Print and shaded views of the part. All mm, measured from the part's lowest x, y and z. Give positions to 0.01 mm unless a question says otherwise; leave off trailing zeros. Order: outer loops, then holes, each group sorted by start corner. A loop starts at its lowest first (then second) coordinate and runs counter-clockwise, first axis right, second up. Notation, with made-up numbers: (15, 78) -> (36, 78) arc R34 ccw to (36, 113) -> close; hole circle Ø11 at (-29, 36). An arc over 180 degrees is marked (long way). One line per question, with ' | ' between items. Start each with the question number.
(1) Cut at B-B (y = 1.35). Give the cut face in (x, z), then the cut area to 3 significant figures.
(2) Cut at A-A (x = 103.5). Give the cut face in (y, z), then the cut area to 4 significant figures.
(3) Cut at C-C (z = 39.5). Give the cut face in (x, y), then the cut area to 4 significant figures.
(4) Pin check, flat tips, straight feed: pin 1 Ø1.1 at (y, z) = (1.5, 19.5) entering from +X; pin 2 Ø0.5 at (x, y) = (96.5, 1.5) entering from -Z; pin 3 Ø0.5 at (y, z) = (1.5, 40.5) entering from -X. Stop position of each tip, or through.
(5) Drill centre lines: L1, parallel to Z at x = 112, y = 1.2; L2, parallel to X at y = 1.55, z = 23.5; L3, parallel to X at y = 0.8, z = 2. Where is each one in solid material? Low to high. Write a range as from..to.
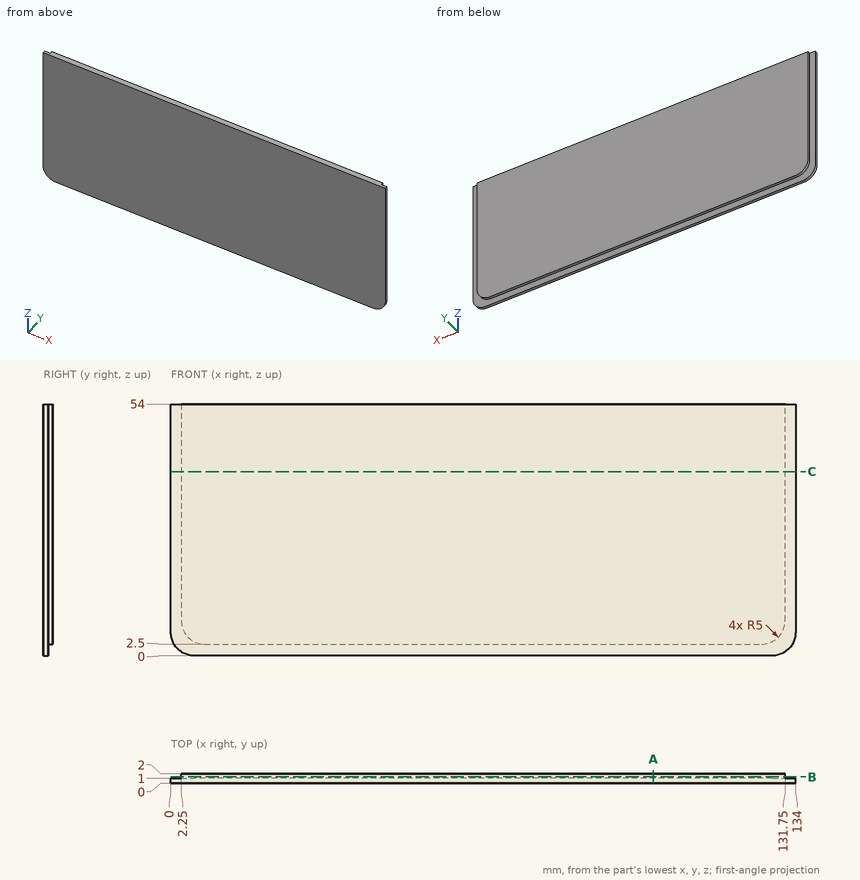
Result set:
1) outline: (2.25, 7.5) arc R5 ccw to (7.25, 2.5) -> (126.75, 2.5) arc R5 ccw to (131.75, 7.5) -> (131.75, 54) -> (2.25, 54) -> close | area: 6,660 mm2
2) outline: (0, 0) -> (1, 0) -> (1, 2.5) -> (2, 2.5) -> (2, 54) -> (0, 54) -> close | area: 105.5 mm2
3) outline: (0, 0) -> (134, 0) -> (134, 1) -> (131.75, 1) -> (131.75, 2) -> (2.25, 2) -> (2.25, 1) -> (0, 1) -> close | area: 263.5 mm2
4) pin 1: stops at x = 134 | pin 2: stops at z = 2.5 | pin 3: stops at x = 2.25
5) L1: z = 2.5..54 | L2: x = 2.25..131.75 | L3: x = 1..133
